from build123d import *

# Parameters (mm, degrees)
CROQUIS1_R              = 3
CROQUIS1_R_2            = 6
SALIENTE_EXTRUIR1_DEPTH = 6


with BuildPart() as part:
    # Croquis1 → Saliente-Extruir1 (new body)
    with BuildSketch(Plane.XY):
        with BuildLine():
            ThreePointArc((0, -6), (2.10674065, -5.617975065), (3.945205479, -4.520547945))
            ThreePointArc((3.945205479, -4.520547945), (5.462198865, -2.482817666), (6, 0))
            ThreePointArc((6, 0), (4.242640687, 4.242640687), (0, 6))
            ThreePointArc((0, 6), (-4.242640687, 4.242640687), (-6, 0))
            ThreePointArc((-6, 0), (-4.242640687, -4.242640687), (0, -6))
        make_face()
        Circle(CROQUIS1_R, mode=Mode.SUBTRACT)
        with BuildLine():
            ThreePointArc((14.287671233, 4.505603985), (15.551832387, 6.203712551), (16, 8.272727273))
            Line((16, 8.272727273), (16, 106.727272727))
            ThreePointArc((16, 106.727272727), (15.677138032, 108.494864262), (14.750248066, 110.034180564))
            Line((14.750248066, 110.034180564), (4.50029768, 121.658289404))
            ThreePointArc((4.50029768, 121.658289404), (5.612565638, 119.811109842), (6, 117.69))
            ThreePointArc((6, 117.69), (4.242640687, 113.447359313), (0, 111.69))
            Line((0, 111.69), (1, 111.69))
            ThreePointArc((1, 111.69), (4.535533906, 110.225533906), (6, 106.69))
            Line((6, 106.69), (6, 11))
            ThreePointArc((6, 11), (4.535533906, 7.464466094), (1, 6))
            Line((1, 6), (0, 6))
            ThreePointArc((0, 6), (4.242640687, 4.242640687), (6, 0))
            ThreePointArc((6, 0), (5.462198865, -2.482817666), (3.945205479, -4.520547945))
            Line((3.945205479, -4.520547945), (14.287671233, 4.505603985))
        make_face()
        with Locations((0, 117.69)):
            Circle(CROQUIS1_R_2)
        with Locations((0, 117.69)):
            Circle(CROQUIS1_R, mode=Mode.SUBTRACT)
    extrude(amount=SALIENTE_EXTRUIR1_DEPTH)


solid = part.part
Model file for the job. Use its own axes, mm. A direction names the side the tool comes from. Round coordinates to 2 decimals unless told otherwise and drop trailing zeros. Order: outer loops, then holes, each group sorted by start corner. A loop starts at its lowest first (then second) coordinate and runs counter-clockwise, first axis right, second up.
(1) Band-saw the part on D-D (y = 84). List the corners of the cut face in (x, z), then the cut area to 3 significant figures.
(2) Band-saw the part on A-A (z = 4.3). List the corners of the cut face in (x, y), then the cut area to 3 significant figures.
(3) Drill centre lines: line 1 (Y direction, x = 0.25, z = 0.35); line 2 (X direction, y = 59, z = 5.4); line 3 (Y direction, x = 5.25, z = 3.65). Where is each one in solid material? Low to high.
(4) Band-saw the part on B-B (y = 117.69). List the corners of the cut face in (x, z), then the cut area to 3 significant figures.
(5) 3-axis set-ups, long thin cutter, end or side, ignore diameter. For faces 4 (the face through (-3, 0, 3)), 5 (the face through (4.5, 110.26, 2.96)): which of +Z, -Z, +X, -X, +Y, -Y reach the whole face in a straight line?
(6) Pin check, flat tips, straight feed: pin 1 (3 mm diameter, centred on y = 78.5, z = 4, fed in from -X); pin 2 (1 mm diameter, centred on x = -1.5, z = 1.5, fed in from +Y); pin 3 (0.5 mm diameter, centred on x = 0.5, z = 4.5, fed in from -Y). Stop position of each tip, or through.
(7) Band-saw the part on C-C (x = 8.75). List the corners of the cut face in (y, z).
(8) Pull direction Y, two halves, no side cores. Call faces 1 (the face through (9.7, 115.76, 2.96)), 2 (the face through (15.54, 6.18, 2.96)), 3 (the face through (-5.397, 120.311, 2.958)): released by +Y, released by -Y, zero draft, split by the parting line, or undercut.
Verdict:
1. outline: (6, 0) - (16, 0) - (16, 6) - (6, 6) - close
1. area: 60.0 mm2
2. outline: (0, 6) arc R6 ccw (long way) to (3.95, -4.52) - (14.29, 4.51) arc R5 ccw to (16, 8.27) - (16, 106.73) arc R5 ccw to (14.75, 110.03) - (4.5, 121.66) arc R6 ccw (long way) to (0, 111.69) - (1, 111.69) arc R5 cw to (6, 106.69) - (6, 11) arc R5 cw to (1, 6) - close; hole circle Ø6 at (0, 0); hole circle Ø6 at (0, 117.69)
2. area: 1,320 mm2
3. line 1: y = -5.99 to -2.99, 2.99 to 6, 111.69 to 114.7, 120.68 to 123.68
3. line 2: x = 6 to 16
3. line 3: y = -3.38 to 8.37, 109.32 to 120.81
4. outline: (-6, 0) - (-3, 0) - (-3, 6) - (-6, 6) - close; (3, 0) - (8, 0) - (8, 6) - (3, 6) - close
4. area: 48.0 mm2
5. face 4: +Z, -Z
5. face 5: +Z, -Z, -X
6. pin 1: stops at x = 6
6. pin 2: stops at y = 123.61
6. pin 3: stops at y = -5.99
7. outline: (-0.33, 0) - (116.84, 0) - (116.84, 6) - (-0.33, 6) - close
8. face 1: released by +Y
8. face 2: released by -Y
8. face 3: undercut
